from build123d import *

# Parameters (mm, degrees)
F0_W      = 11.41
F0_H      = 15.49
F1_DEPTH  = 1.39
F2_W      = 8.48
F2_H      = 14.17
F3_DEPTH  = 1
F4_R      = 3.23
F5_DEPTH  = 9.16
F6_R      = 4
F7_R      = 2.809954
F8_DEPTH  = 11.551
F10_DEPTH = 25
F12_DEPTH = 1.87


with BuildPart() as f1:
    # F0 (on Front) → F1 (new body)
    with BuildSketch(Plane.XZ):
        with Locations((1.059828, 4.585434)):
            Rectangle(F0_W, F0_H)
    extrude(amount=F1_DEPTH)

    # F2 (on face) → F3 (join)
    with BuildSketch(Plane.XZ.offset(1.39)):
        with Locations((1.059828, 3.925434)):
            Rectangle(F2_W, F2_H)
    extrude(amount=F3_DEPTH)

    # F4 (on face) → F5 (join)
    with BuildSketch(Plane.XZ.offset(2.39)):
        with Locations((1.059828, 6.640434)):
            Circle(F4_R)
    extrude(amount=F5_DEPTH)

    # F6
    f6_edges = [f1.edges().sort_by_distance(p)[0] for p in [
        (-4.645172, -0.695, 12.330434),
        (6.764828, -0.695, 12.330434),
        (5.299828, -1.89, 11.010434),
        (-3.180172, -1.89, 11.010434),
    ]]
    fillet(f6_edges, radius=F6_R)

    # F7 (on Front) → F8 (cut, through all)
    with BuildSketch(Plane.XZ):
        with Locations((1.043937, 6.664116)):
            Circle(F7_R)
    extrude(amount=F8_DEPTH, mode=Mode.SUBTRACT)

    # F9 (on Top) → F10 (cut)
    with BuildSketch(Plane.XY):
        Polygon((5.4795, -12.259658), (-2.155284, -7.637704), (-4.158131, -12.259658), align=None)
    extrude(amount=F10_DEPTH, mode=Mode.SUBTRACT)

    # F11 (on face) → F12 (cut)
    with BuildSketch(Plane.XZ.offset(2.39)):
        with BuildLine():
            ThreePointArc((4.179828, 2.253996), (1.059828, 0.2656), (-2.060172, 2.253996))
            Line((-2.060172, 2.253996), (-2.060172, -2.769004))
            Line((-2.060172, -2.769004), (4.179828, -2.769004))
            Line((4.179828, -2.769004), (4.179828, 2.253996))
        make_face()
    extrude(amount=-F12_DEPTH, mode=Mode.SUBTRACT)


solid = f1.part
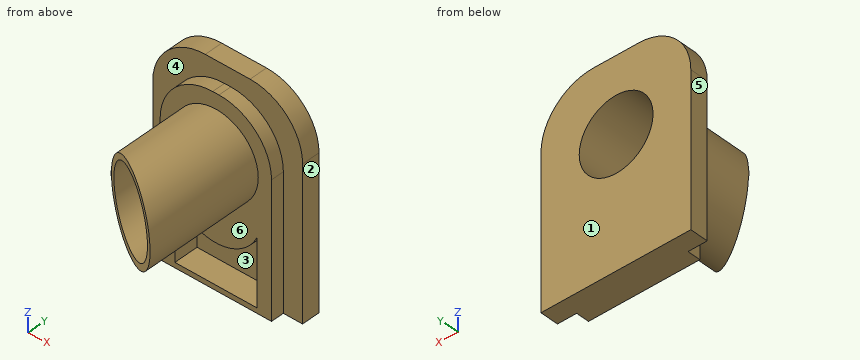
Verification items for the finished model (mm, model axes). Face numbers are marked on the shaded views. A direction names the side the tool comes from. Coordinates: 2 decimals unless noted, no trailing zeros. Loops run counter-clockwise (first coordinate to the right, second up) from the corner with the lowest first, then second, coordinate; pieces in that order, holes last. Notation, with made-up numbers: (47.5, 84) -> (64.5, 84) arc R22 ccw to (64.5, 108) -> close; hole circle Ø8 at (86.25, 9). An arc over 180 degrees is marked (long way). Answer as CSV lines item,"result".
1) Tool access check on the marked faces 4, 5 and 6. Record the directions out of +Z, -Z, +X, -X, +Y, -Y that give a thin tool (end or side, any length) a straight path to the whole face; none if there is none.
Found:
face 4,"+Z, -Y"
face 5,"+Z, -Z, -X, +Y, -Y"
face 6,"-Y"
2) Cross-section at B-B, the plane x = -1.5. Record the cut outline in (y, z), then the cut area to 3 significant figures.
Found:
outline,"(-8.03, 4.67) -> (-2.39, 4.67) -> (-2.39, 1.41) -> (-0.52, 1.41) -> (-0.52, -2.77) -> (-2.39, -2.77) -> (-2.39, -3.16) -> (0, -3.16) -> (0, 5.47) -> (-8.03, 5.47) -> close; (-8.03, 7.86) -> (0, 7.86) -> (0, 12.24) -> (-1.39, 12.24) -> (-1.39, 10.27) -> (-2.39, 10.27) -> (-2.39, 8.61) -> (-8.03, 8.61) -> close"
area,"30.1 mm2"
3) Depth check by flat-ended pin: pin 1 (3.5 mm diameter, centred on x = 1.04, z = 6.66, fed in from +Y); pin 2 (4 mm diameter, centred on x = 1.5, z = 0.5, fed in from -Y); pin 3 (6 mm diameter, centred on y = -4, z = 10.5, fed in from +X); pin 4 (0.8 mm diameter, centred on y = -2, z = 4, fed in from -X). Enter the tip coordinate at first touch or a pass-through.
Found:
pin 1,"passes through"
pin 2,"stops at y = -2.39"
pin 3,"stops at x = 6.7"
pin 4,"stops at x = -3.18"
4) Cross-section at D-D, the plane y = -2. Record the cut outline in (x, z).
Found:
outline,"(-3.18, -3.16) -> (5.3, -3.16) -> (5.3, 7.01) arc R4 ccw to (1.3, 11.01) -> (0.82, 11.01) arc R4 ccw to (-3.18, 7.01) -> close; hole (-2.06, -2.77) -> (4.18, -2.77) -> (4.18, 2.25) arc R3.44 cw to (-2.06, 2.25) -> close; hole circle Ø5.62 at (1.04, 6.66)"
5) Release check for a two-part mould opening along X. For the marked faces 1, 2 and 3 record: +X half, -X half, draft (parallel to the pull), parting line (faces both ways), or undercut.
Found:
face 1,"draft"
face 2,"+X half"
face 3,"undercut"
6) Cross-section at C-C, the plane z = 9.25. Record the cut outline in (x, y).
Found:
outline,"(-4.54, -1.39) -> (-2.49, -1.39) -> (-2.49, -2.39) -> (-0.84, -2.39) -> (-0.84, -8.43) -> (-0.06, -8.91) -> (-0.06, 0) -> (-4.54, 0) -> close; (2.14, -10.24) -> (2.96, -10.74) -> (2.96, -2.39) -> (4.61, -2.39) -> (4.61, -1.39) -> (6.66, -1.39) -> (6.66, 0) -> (2.14, 0) -> close"
7) Thickness scan on L1, parallel to Z at x = -0.25, y = -1.75; L2, parallel to Y at x = -0.5, z = 3.5; L3, parallel to X at y = -2, z = 0. Record the ranges inside material, lowest first. Write a range as from..to.
Found:
L1,"z = -3.16..-2.77, 0.52..4.17, 9.16..10.86"
L2,"y = -2.39..0"
L3,"x = -3.18..-2.06, 4.18..5.3"
8) Cross-section at A-A, the plane z = 2.5. Record the cut outline in (x, y).
Found:
outline,"(-4.65, -1.39) -> (-3.18, -1.39) -> (-3.18, -2.39) -> (5.3, -2.39) -> (5.3, -1.39) -> (6.76, -1.39) -> (6.76, 0) -> (-4.65, 0) -> close"
